```python
from build123d import *

# Parameters (mm, degrees)
BOSS_EXTRUDE1_DEPTH = 28
CUT_EXTRUDE1_START  = 28
CUT_EXTRUDE1_DEPTH  = 10
BOSS_EXTRUDE2_START = -10
SKETCH5_R           = 3
BOSS_EXTRUDE2_DEPTH = 6


with BuildPart() as part:
    # Sketch2 → Boss-Extrude1 (new body)
    with BuildSketch(Plane.YZ):
        Polygon((0, 0), (78, 0), (78, 44.523418625), (67.909286037, 49.228795822), (52.695028614, 16.601715489), (47.695028614, 18.933253779), (62.909286037, 51.560334113), (49.099377976, 58), (40, 38.486320959), (24, 38.486320959), (24, 16), (0, 16), (0, 8), align=None)
    extrude(amount=BOSS_EXTRUDE1_DEPTH)

    # Sketch3 → Cut-Extrude1 (cut)
    with BuildSketch(Plane.YZ.offset(CUT_EXTRUDE1_START)):
        Polygon((0, 8), (0, 16), (24, 16), (24, 38.486320959), (40, 38.486320959), (24, 8), align=None)
    extrude(amount=-CUT_EXTRUDE1_DEPTH, mode=Mode.SUBTRACT)

    # Sketch5 → Boss-Extrude2 (add)
    with BuildSketch(Plane(origin=(0, 35.210924553, 75.510071381), x_dir=(1, 0, 0), z_dir=(0, 0.42261826174070044, 0.9063077870366496)).offset(BOSS_EXTRUDE2_START)):
        with Locations(Location((7, 27.487289417, 0), (0, 0, 90))):
            Circle(SKETCH5_R)
        with Locations(Location((21, 27.487289417, 0), (0, 0, 90))):
            Circle(SKETCH5_R)
    extrude(amount=BOSS_EXTRUDE2_DEPTH)


solid = part.part
```
Source: CAD feature listing. Evaluate the final solid. Frame: model axes, mm. A direction names the side the tool comes from. Give positions to 0.01 mm unless a question says otherwise; leave off trailing zeros. Write each loop counter-clockwise with the first axis right and the second up, starting at its lowest first coordinate (ties: lowest second). Pieces come first, ordered by that corner, then holes.
1. Pull-direction query (X, two-part tool) for faces 1 (the face through (18, 25, 23)), 2 (the face through (4.972, 55.143, 58.446)), 3 (the face through (13.804, 56.101, 54.735)), 4 (the face through (13.804, 60.409, 33.144)); classes: +X half, -X half, draft (parallel to the pull), parting line (faces both ways), or undercut.
2. Section query A-A (x = 15). Return the cut outline in (y, z).
3. First-contact query: pin 1 (5 mm diameter, centred on x = 7.5, z = 36.5, fed in from -Y); pin 2 (3 mm diameter, centred on x = 7.5, y = 14.5, fed in from +Z); pin 3 (1 mm diameter, centred on x = 23.5, y = 11, fed in from +Z). Flat tips, straight axial feed; report the tip coordinate or a pass-through.
4. Section query C-C (z = 29). Return the cut outline in (x, y), then the cut area to 3 significant figures.
5. Material intervals for line 1 along Y through (x, z) = (9.5, 28); line 2 along X through (y, z) = (10.5, 14); line 3 along Z through (x, y) = (25.5, 62), sorted ascending.
6. Access query for faces 5 (the face through (23.07, 32.112, 23.457)), 6 (the face through (13.8, 50.23, 17.75)), 7 (the face through (9, 32, 38.486)). Directions: +Z, -Z, +X, -X, +Y, -Y. A direction counts if a zero-diameter tool reaches every point of the face in a straight line with its end or side. Return the directions, or none.
7. Section query D-D (x = 23). Return the cut outline in (y, z).
8. Section query B-B (y = 6). Return the cut outline in (x, z), then the cut area to 3 significant figures.
Output values:
1. face 1: +X half
1. face 2: undercut
1. face 3: undercut
1. face 4: draft
2. outline: (0, 0) - (78, 0) - (78, 44.52) - (67.91, 49.23) - (52.7, 16.6) - (47.7, 18.93) - (62.91, 51.56) - (49.1, 58) - (40, 38.49) - (24, 38.49) - (24, 16) - (0, 16) - close
3. pin 1: stops at y = 24
3. pin 2: stops at z = 16
3. pin 3: stops at z = 8
4. outline: (0, 24) - (18, 24) - (18, 35.02) - (28, 35.02) - (28, 52.39) - (0, 52.39) - close; (0, 58.48) - (28, 58.48) - (28, 78) - (0, 78) - close
4. area: 1,230 mm2
5. line 1: y = 24 to 51.92, 58.01 to 78
5. line 2: x = 0 to 18
5. line 3: z = 0 to 36.56, 49.61 to 51.98
6. face 5: +Z, +X, -Y
6. face 6: +X, -X
6. face 7: +Z, +X, -X, -Y
7. outline: (0, 0) - (78, 0) - (78, 44.52) - (67.91, 49.23) - (52.7, 16.6) - (47.7, 18.93) - (62.91, 51.56) - (57.92, 53.89) - (60.46, 59.32) - (56.41, 61.21) - (53.87, 55.78) - (49.1, 58) - (40, 38.49) - (24, 8) - (0, 8) - close
8. outline: (0, 0) - (28, 0) - (28, 8) - (18, 8) - (18, 16) - (0, 16) - close
8. area: 368 mm2
